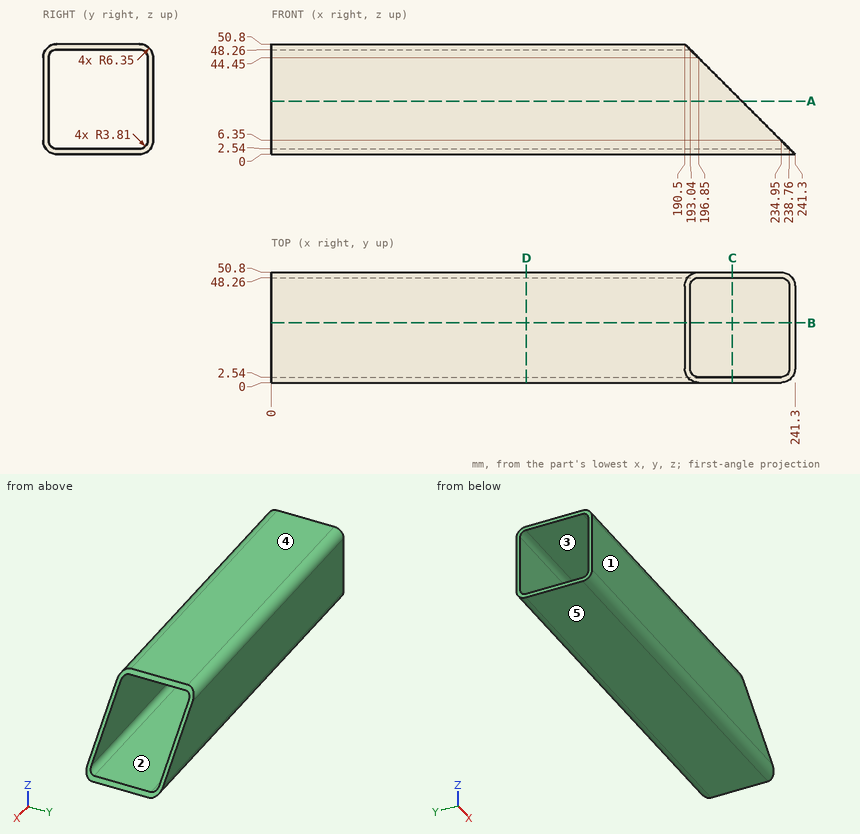
Print and shaded views of the part. All mm, measured from the part's lowest x, y and z. A direction names the side the tool comes from. Coordinates: 2 decimals unless noted, no trailing zeros. Order: outer loops, then holes, each group sorted by start corner. A loop starts at its lowest first (then second) coordinate and runs counter-clockwise, first axis right, second up. Notation, with made-up numbers: M 10,-6.5 L 17,-6.5 A21 cw 17,7.5 Z; hole C 19.25,34 d3. An arc over 180 degrees is marked long. One line per question, with ' | ' between items. Start each with the question number.
Q1. 3-axis set-ups, long thin cutter, end or side, ignore diameter. For the marked faces 1 and 2: which of +Z, -Z, +X, -X, +Y, -Y reach the whole face in a straight line?
Q2. Two-plate mould, pull along Z, no slides. Class the marked faces 3, 4 and 5: +Z half, -Z half, draft (parallel to the pull), parting line (faces both ways), or undercut.
Q3. Saw through at C-C (x = 212.5). List the corners of the cut face in (y, z), then the cut area to 3 significant figures.
Q4. Probe L1, parallel to Y at x = 41.5, z = 39; L2, parallel to Z at x = 189, y = 45.5. List the from-to ranges inside material, lowest first. Write a range as from..to.
Q5. Saw through at A-A (z = 24.5). List the corners of the cut face in (x, y).
Q6. Saw through at D-D (x = 117.5). List the corners of the cut face in (y, z), then the cut area to 3 significant figures.
Q7. Saw through at B-B (y = 27.5). List the corners of the cut face in (x, z), then the cut area to 3 significant figures.
Q8. Flat gauge pin, fed straight in: pin 1 Ø10 at (y, z) = (39, 16.5) entering from -X. Where does the tip first touch, or does it go through?
Check values:
1) face 1: +Z, -Z, +X, -X, -Y | face 2: +X, -X
2) face 3: undercut | face 4: +Z half | face 5: -Z half
3) outline: M 0,6.35 A6.35 ccw 6.35,0 L 44.45,0 A6.35 ccw 50.8,6.35 L 50.8,28.8 L 48.26,28.8 L 48.26,6.35 A3.81 cw 44.45,2.54 L 6.35,2.54 A3.81 cw 2.54,6.35 L 2.54,28.8 L 0,28.8 Z | area: 251 mm2
4) L1: y = 0..2.54, 48.26..50.8 | L2: z = 0.09..2.69, 48.11..50.71
5) outline: M 0,0 L 216.8,0 L 216.8,2.54 L 0,2.54 Z; M 0,48.26 L 216.8,48.26 L 216.8,50.8 L 0,50.8 Z
6) outline: M 0,6.35 A6.35 ccw 6.35,0 L 44.45,0 A6.35 ccw 50.8,6.35 L 50.8,44.45 A6.35 ccw 44.45,50.8 L 6.35,50.8 A6.35 ccw 0,44.45 Z; hole M 2.54,6.35 A3.81 ccw 6.35,2.54 L 44.45,2.54 A3.81 ccw 48.26,6.35 L 48.26,44.45 A3.81 ccw 44.45,48.26 L 6.35,48.26 A3.81 ccw 2.54,44.45 Z | area: 468 mm2
7) outline: M 0,0 L 241.3,0 L 238.76,2.54 L 0,2.54 Z; M 0,48.26 L 193.04,48.26 L 190.5,50.8 L 0,50.8 Z | area: 1,100 mm2
8) pin 1: passes through
